Source: CAD feature listing. Evaluate the final solid. Frame: model axes, mm. A direction names the side the tool comes from. Give positions to 0.01 mm unless a question says otherwise; leave off trailing zeros. Order: outer loops, then holes, each group sorted by start corner. A loop starts at its lowest first (then second) coordinate and runs counter-clockwise, first axis right, second up.
```python
from build123d import *

# Parameters (mm, degrees)
SKETCH1_R           = 2
BOSS_EXTRUDE1_DEPTH = 10
CUT_EXTRUDE1_DEPTH  = 11


with BuildPart() as part:
    # Sketch1 → Boss-Extrude1 (new body)
    with BuildSketch(Plane(origin=(0, 0, 0), x_dir=(1, 0, 0), z_dir=(0, 1, 0))):
        with BuildLine():
            Line((0.090909042, -11.49964067), (280.070567987, -9.286294776))
            ThreePointArc((280.070567987, -9.286294776), (289.991484188, 0.738871766), (280.019610714, 10.7133533))
            Line((280.019610714, 10.7133533), (0.032308177, 11.499954617))
            ThreePointArc((0.032308177, 11.499954617), (-11.499962672, -0.029300853), (0.090909042, -11.49964067))
        make_face()
        with Locations((250, 0)):
            Circle(SKETCH1_R, mode=Mode.SUBTRACT)
        Circle(SKETCH1_R, mode=Mode.SUBTRACT)
    extrude(amount=BOSS_EXTRUDE1_DEPTH)

    # Sketch2 → Cut-Extrude1 (cut, through all)
    with BuildSketch(Plane(origin=(0, 10, 0), x_dir=(1, 0, 0), z_dir=(0, 1, 0))):
        with BuildLine():
            Line((17.967691823, 6.449546898), (116.670959066, 6.17224818))
            ThreePointArc((116.670959066, 6.17224818), (122.825891181, 0), (116.670959066, -6.17224818))
            Line((116.670959066, -6.17224818), (17.967691823, -6.449546898))
            ThreePointArc((17.967691823, -6.449546898), (11.5, 0), (17.967691823, 6.449546898))
        make_face()
        with BuildLine():
            Line((133.966776262, 6.123657003), (232.670043506, 5.846358285))
            ThreePointArc((232.670043506, 5.846358285), (238.5, 0), (232.670043506, -5.846358285))
            Line((232.670043506, -5.846358285), (133.966776262, -6.123657003))
            ThreePointArc((133.966776262, -6.123657003), (127.825891181, 0), (133.966776262, 6.123657003))
        make_face()
    extrude(amount=-CUT_EXTRUDE1_DEPTH, mode=Mode.SUBTRACT)


solid = part.part
```
1) Reachability of faces 4 (the flat face through (137, 0, -8)), 5 (the cylindrical face through (11.5, 5.1, 0.1)) from +Z, -Z, +X, -X, +Y, -Y: full face, straight path, thin tool, end or side. Return the list, or none.
Report:
face 4: +Z, -Z, +X, -X, -Y
face 5: +Y, -Y
2) Section query B-B, the plane x = 44. Return the cut outline in (y, z), and give its area (3 significant figures).
Report:
outline: (0, -11.38) - (10, -11.38) - (10, -6.38) - (0, -6.38) - close; (0, 6.38) - (10, 6.38) - (10, 11.15) - (0, 11.15) - close
area: 97.8 mm2
3) Material intervals for L1, parallel to X at y = 8.25, z = 0; L2, parallel to X at y = 6.75, z = 4; L3, parallel to X at y = 9, z = 4.25, sorted ascending.
Report:
L1: x = -11.5 to -2, 2 to 11.5, 122.83 to 127.83, 238.5 to 248, 252 to 289.97
L2: x = -10.78 to 12.89, 121.35 to 129.31, 236.92 to 288.81
L3: x = -10.69 to 13.1, 121.13 to 129.54, 236.67 to 288.67
4) Draft query along Z for faces 1 (the cylindrical face through (-11.5, 4.9, -0.2)), 2 (the cylindrical face through (122.824, 5.07, -0.135)), 3 (the flat face through (137, 10, -8)). Return one class per face: +Z half, -Z half, draft (parallel to the pull), parting line (faces both ways), or undercut.
Report:
face 1: parting line
face 2: undercut
face 3: draft
5) Pin query (flat end, axial travel): pin 1 (8 mm diameter, centred on x = 26.5, z = 4.5, fed in from -Y); pin 2 (2 mm diameter, centred on x = 99, y = 8.5, fed in from -Z); pin 3 (4 mm diameter, centred on x = 95, y = 3, fed in from +Z); pin 4 (4 mm diameter, centred on x = 53, y = 4, fed in from -Z). Return the tip coordinate at first contact, or that it passes through.
Report:
pin 1: stops at y = 0
pin 2: stops at z = -11.22
pin 3: stops at z = 10.77
pin 4: stops at z = -11.36
6) Section query A-A, the plane y = 4. Return the cut outline in (x, z), and give its area (3 significant figures).
Report:
outline: (0.03, -11.5) - (280.02, -10.71) arc R10 ccw to (280.07, 9.29) - (0.09, 11.5) arc R11.5 ccw (long way) to start; hole circle Ø4 at (0, 0); hole (17.97, -6.45) - (116.67, -6.17) arc R6.17 ccw to (116.67, 6.17) - (17.97, 6.45) arc R6.45 ccw (long way) to start; hole (133.97, -6.12) - (232.67, -5.85) arc R5.85 ccw to (232.67, 5.85) - (133.97, 6.12) arc R6.12 ccw (long way) to start; hole circle Ø4 at (250, 0)
area: 3,690 mm2
